from build123d import *

# Parameters (mm, degrees)
HOLE_TOPMAIN_OUTLINE_W = 12.9
HOLE_TOPMAIN_OUTLINE_H = 12.9
HOLE_TOPMAIN_OUTLINE_R = 2.5
HOLE_TOPMAIN_DEPTH     = 64.27
SKETCH14_R             = 2.5
CUT_EXTRUDE9_DEPTH     = 67.100627077
SKETCH15_R             = 3.25
CUT_EXTRUDE10_DEPTH    = 66.309210028
SKETCH18_W             = 12.9
SKETCH18_H             = 64.27
SKETCH18_R             = 3.25
BOSS_EXTRUDE2_DEPTH    = 13.5
FILLET3_R              = 2
SKETCH19_R             = 2.5
CUT_EXTRUDE11_DEPTH    = 13.5
SKETCH22_W             = 13.5
SKETCH22_H             = 64.27
BOSS_EXTRUDE3_DEPTH    = 13.5
BOSS_EXTRUDE5_START    = -26.4
SKETCH24_R             = 3.25
BOSS_EXTRUDE5_DEPTH    = 26.4
CUT_EXTRUDE12_START    = -64.27
SKETCH25_R             = 2.5
CUT_EXTRUDE12_DEPTH    = 64.27
SKETCH26_R             = 2.5
CUT_EXTRUDE13_DEPTH    = 13.5
SKETCH28_R             = 2.5
CUT_EXTRUDE14_DEPTH    = 13.5
FILLET4_R              = 2
SKETCH29_W             = 0.2
SKETCH29_H             = 25.271779789
CUT_EXTRUDE15_DEPTH    = 64.27


# Read off the part's stored shape, not the designer's step: hole-TopMain
with BuildPart() as part:
    # hole-TopMain outline → hole-TopMain (new body)
    with BuildSketch(Plane(origin=(0, 0, 0), x_dir=(1, 0, 0), z_dir=(0, 1, 0))):
        with Locations((-2.05, 2.05)):
            Rectangle(HOLE_TOPMAIN_OUTLINE_W, HOLE_TOPMAIN_OUTLINE_H)
        Circle(HOLE_TOPMAIN_OUTLINE_R, mode=Mode.SUBTRACT)
    extrude(amount=HOLE_TOPMAIN_DEPTH)

    # Sketch14 → Cut-Extrude9 (cut, through all)
    with BuildSketch(Plane(origin=(0, 0, -8.5), x_dir=(-1, 0, 0), z_dir=(0, 0, -1))):
        with Locations((1.75, 46.135)):
            Circle(SKETCH14_R)
    extrude(amount=-CUT_EXTRUDE9_DEPTH, mode=Mode.SUBTRACT)

    # Sketch15 → Cut-Extrude10 (cut, through all)
    with BuildSketch(Plane(origin=(0, 0, -3.5), x_dir=(-1, 0, 0), z_dir=(0, 0, -1))):
        with Locations((1.75, 46.135)):
            Circle(SKETCH15_R)
    extrude(amount=-CUT_EXTRUDE10_DEPTH, mode=Mode.SUBTRACT)

    # Sketch18 → Boss-Extrude2 (add)
    with BuildSketch(Plane.XY.offset(4.4)):
        with Locations((-2.05, 32.135)):
            Rectangle(SKETCH18_W, SKETCH18_H)
        with Locations(Location((-1.75, 46.135, 0), (0, 0, 180))):
            Circle(SKETCH18_R, mode=Mode.SUBTRACT)
    extrude(amount=BOSS_EXTRUDE2_DEPTH)

    # Fillet3
    fillet3_edges = [part.edges().sort_by_distance(p)[0] for p in [
        (-8.5, 32.135, -8.5),
        (4.4, 32.135, 17.9),
    ]]
    fillet(fillet3_edges, radius=FILLET3_R)

    # Sketch19 → Cut-Extrude11 (cut)
    with BuildSketch(Plane.ZY.offset(8.5)):
        with Locations((11.55, 46.135)):
            Circle(SKETCH19_R)
    extrude(amount=-CUT_EXTRUDE11_DEPTH, mode=Mode.SUBTRACT)

    # Sketch22 → Boss-Extrude3 (add)
    with BuildSketch(Plane(origin=(4.4, 0, 0), x_dir=(0, 0, -1), z_dir=(1, 0, 0))):
        with Locations((1.75, 32.135)):
            Rectangle(SKETCH22_W, SKETCH22_H)
    extrude(amount=BOSS_EXTRUDE3_DEPTH)

    # Sketch24 → Boss-Extrude5 (add)
    with BuildSketch(Plane.XY.offset(17.9).offset(BOSS_EXTRUDE5_START)):
        with Locations((-1.75, 46.135)):
            Circle(SKETCH24_R)
    extrude(amount=BOSS_EXTRUDE5_DEPTH)

    # Sketch25 → Cut-Extrude12 (cut)
    with BuildSketch(Plane(origin=(0, 64.27, 0), x_dir=(1, 0, 0), z_dir=(0, 1, 0)).offset(CUT_EXTRUDE12_START)):
        with Locations(Location((0, 0, 0), (0, 0, 90))):
            Circle(SKETCH25_R)
    extrude(amount=CUT_EXTRUDE12_DEPTH, mode=Mode.SUBTRACT)

    # Sketch26 → Cut-Extrude13 (cut)
    with BuildSketch(Plane.ZY.offset(8.5)):
        with Locations((11.55, 46.135)):
            Circle(SKETCH26_R)
    extrude(amount=-CUT_EXTRUDE13_DEPTH, mode=Mode.SUBTRACT)

    # Sketch28 → Cut-Extrude14 (cut)
    with BuildSketch(Plane(origin=(0, 0, -8.5), x_dir=(-1, 0, 0), z_dir=(0, 0, -1))):
        with Locations((-11.35, 46.135)):
            Circle(SKETCH28_R)
    extrude(amount=-CUT_EXTRUDE14_DEPTH, mode=Mode.SUBTRACT)

    # Fillet4
    fillet4_edges = [part.edges().sort_by_distance(p)[0] for p in [
        (17.9, 32.135, 5),
    ]]
    fillet(fillet4_edges, radius=FILLET4_R)

    # Sketch29 → Cut-Extrude15 (cut)
    with BuildSketch(Plane(origin=(0, 64.27, 0), x_dir=(1, 0, 0), z_dir=(0, 1, 0))):
        with Locations((-8.4, -5.264110106)):
            Rectangle(SKETCH29_W, SKETCH29_H)
    extrude(amount=-CUT_EXTRUDE15_DEPTH, mode=Mode.SUBTRACT)


solid = part.part
Design review of the part built by this model. Coordinates are the model's own, in mm. A direction names the side the tool comes from. Give positions to 0.01 mm unless a question says otherwise; leave off trailing zeros. Write each loop counter-clockwise with the first axis right and the second up, starting at its lowest first coordinate (ties: lowest second). Pieces come first, ordered by that corner, then holes. Notation, with made-up numbers: M 63.5,88 L 105.5,88 A20 ccw 105.5,104 Z; hole C 82,-28 d3. An arc over 180 degrees is marked long. Answer as a JSON object with one key per item and string values. Group by question number.
1) Mouldability with a two-part tool opening along X and no side actions: class faces 3 (the face through (-0.54, 31.69, 2.44)), 4 (the face through (10.006, 48.243, -1.844)), 5 (the face through (2, 0, 2)), 6 (the face through (17.9, 33, -3)) as released by +X, released by -X, zero draft, split by the parting line, or undercut.
2) Tool access review of faces 1 (the face through (10, 32, 5)), 2 (the face through (-8.3, 33, 5)): name each direction out of +Z, -Z, +X, -X, +Y, -Y from which nothing blocks a thin tool from reaching the whole face with its end or side.
3) For line 1 along Y through (x, z) = (11.35, -3) (3 decimals); line 2 along X through (y, z) = (28.5, 0); line 3 along Z through (x, y) = (0, 33), list the stretches that pass through material, from the lowest coordinate up.
4) We need section D-D (z = 0). Give the boundary of the cut face in (x, y) (3 decimals), and give its area (3 significant figures).
5) We need section A-A (x = 11.35). Give the boundary of the cut face in (y, z) (3 decimals).
6) We need section C-C (y = 11). Give the boundary of the cut face in (x, z).
7) Clearance check with flat-ended pins moving along their axes: pin 1 Ø5.5 at (x, y) = (12, 33) entering from +Z; pin 2 Ø6.5 at (y, z) = (46.135, 11.55) entering from +X. State where each tip first meets the part, or that it passes through.
8) We need section B-B (z = 11.55). Give the boundary of the cut face in (x, y) (3 decimals).
Answer key:
{
 "1": {"face 3": "undercut", "face 4": "undercut", "face 5": "zero draft", "face 6": "released by +X"},
 "2": {"face 1": "+Z, +X, +Y, -Y", "face 2": "+Z, -Z, -X, +Y, -Y"},
 "3": {"line 1": "y = 0 to 43.635, 48.635 to 64.27", "line 2": "x = -8.3 to -2.5, 2.5 to 17.9", "line 3": "z = -8.5 to -2.5, 2.5 to 17.9"},
 "4": {"outline": "M -8.3,0 L -2.5,0 L -2.5,64.27 L -8.3,64.27 Z; M 2.5,0 L 17.9,0 L 17.9,64.27 L 2.5,64.27 Z; hole C 11.35,46.135 d5", "area": "1,340 mm²"},
 "5": {"outline": "M 0,-8.5 L 43.635,-8.5 L 43.635,5 L 0,5 Z; M 48.635,-8.5 L 64.27,-8.5 L 64.27,5 L 48.635,5 Z"},
 "6": {"outline": "M -8.3,-7.37 A2 ccw -6.5,-8.5 L 17.9,-8.5 L 17.9,3 A2 ccw 15.9,5 L 4.4,5 L 4.4,15.9 A2 ccw 2.4,17.9 L -8.3,17.9 Z; hole C 0,0 d5"},
 "7": {"pin 1": "stops at z = 5", "pin 2": "stops at x = 4.4"},
 "8": {"outline": "M -8.3,0 L 4.4,0 L 4.4,43.635 L -8.3,43.635 Z; M -8.3,48.635 L 4.4,48.635 L 4.4,64.27 L -8.3,64.27 Z"}
}
